from build123d import *

# Parameters (mm, degrees)
BOSS_EXTRUDE1_DEPTH       = 18
F_5_0MM_DOWEL_HOLE1_D     = 5
F_5_0MM_DOWEL_HOLE1_DEPTH = 3
F_5_0MM_DOWEL_HOLE1_TIP   = 1.502151548
FILLET1_R                 = 5
M3_CLEARANCE_HOLE1_D      = 3.6


with BuildPart() as part:
    # Sketch1 → Boss-Extrude1 (new body)
    with BuildSketch(Plane(origin=(0, 0, 0), x_dir=(0, 0, -1), z_dir=(1, 0, 0))):
        Polygon((0, 0), (28.1, 0), (28.1, 3), (3, 3), (3, 13), (0, 13), align=None)
    extrude(amount=BOSS_EXTRUDE1_DEPTH)

    # Ø5.0mm Dowel Hole1
    with Locations(Plane.XY):
        with Locations((9, 8)):
            Hole(F_5_0MM_DOWEL_HOLE1_D / 2, depth=F_5_0MM_DOWEL_HOLE1_DEPTH)
            with Locations((0, 0, -(F_5_0MM_DOWEL_HOLE1_DEPTH + F_5_0MM_DOWEL_HOLE1_TIP / 2))):  # 118° drill point
                Cone(0, F_5_0MM_DOWEL_HOLE1_D / 2, F_5_0MM_DOWEL_HOLE1_TIP, mode=Mode.SUBTRACT)

    # Fillet1
    fillet1_edges = [part.edges().sort_by_distance(p)[0] for p in [
        (18, 13, -1.5),
        (0, 13, -1.5),
    ]]
    fillet(fillet1_edges, radius=FILLET1_R)

    # M3 Clearance Hole1 (through all)
    with Locations(Plane(origin=(0, 3, 0), x_dir=(1, 0, 0), z_dir=(0, 1, 0))):
        with Locations((14, 24.6), (4, 24.6), (4, 14.6), (14, 14.6)):
            Hole(M3_CLEARANCE_HOLE1_D / 2)


solid = part.part
Work out the finished part from the listing and answer in its coordinate system (mm). A direction names the side the tool comes from. Coordinates: 2 decimals unless noted, no trailing zeros. Write each loop counter-clockwise with the first axis right and the second up, starting at its lowest first coordinate (ties: lowest second). Pieces come first, ordered by that corner, then holes. Notation, with made-up numbers: M 30.5,-29.5 L 86.5,-29.5 A14 cw 86.5,-8.5 Z; hole C 74,2 d4. An arc over 180 degrees is marked long. Use one line per item in the form item = value. Start each with the question number.
1. Each of these flat-tipped pins is pushed along its axis until it touches: P1, Ø5, axis at x = 7.5, y = 10.5, coming from the -Z side; P2, Ø2, axis at x = 13.5, z = -24.5, coming from the +Y side; P3, Ø6, axis at x = 14, z = -7.5, coming from the +Y side. Where does it stop, or does it pass through?
2. A tool of negligible diameter and unlimited length cuts with its end or side. For faces 1 (the face through (9, 3, -16)), 2 (the face through (18, 2, -11)), from which of +Z, -Z, +X, -X, +Y, -Y can it reach the whole face along a straight path? Write none if from no direction.
3. The mould has two halves that part along X. Classify faces 3 (the face through (3.169, 1.479, -23.003)), 4 (the face through (2, 12, -1)), 5 (the face through (9, 0, -14)): released by +X, released by -X, zero draft, split by the parting line, or undercut.
4. The part is cut by section C-C (x = 4). Give the vertices of the cut face in (y, z).
5. The part is cut by section D-D (y = 3.5). Give the vertices of the cut face in (x, z).
6. The part is cut by section B-B (x = 9). Give the vertices of the cut face in (y, z).
7. The part is cut by section A-A (z = -24.6). Give the vertices of the cut face in (x, y), plus the area to 3 significant figures.
8. Straight lines are drawn through the part: probe 1 along Z at (x, y) = (14, 0.65); probe 2 along X at (y, z) = (1.5, -24.6); probe 3 along Y at (x, z) = (13.25, -7). For each, find the intervals that lie inside material, in ascending order. Write a range as from..to.
Evaluation:
q1.P1 = -3
q1.P2 = through
q1.P3 = 3
q2.face_1 = -Z, +X, -X, +Y
q2.face_2 = +Z, -Z, +X, +Y, -Y
q3.face_3 = undercut
q3.face_4 = released by -X
q3.face_5 = zero draft
q4.outline = M 0,-28.1 L 3,-28.1 L 3,-26.4 L 0,-26.4 Z; M 0,-22.8 L 3,-22.8 L 3,-16.4 L 0,-16.4 Z; M 0,-12.8 L 3,-12.8 L 3,-3 L 12.9,-3 L 12.9,0 L 0,0 Z
q5.outline = M 0,-3 L 18,-3 L 18,0 L 0,0 Z
q6.outline = M 0,-28.1 L 3,-28.1 L 3,-3 L 5.5,-3 L 5.5,0 L 0,0 Z; M 10.5,-3 L 13,-3 L 13,0 L 10.5,0 Z
q7.outline = M 0,0 L 2.2,0 L 2.2,3 L 0,3 Z; M 5.8,0 L 12.2,0 L 12.2,3 L 5.8,3 Z; M 15.8,0 L 18,0 L 18,3 L 15.8,3 Z
q7.area = 32.4 mm^2
q8.probe_1 = -28.1..-26.4, -22.8..-16.4, -12.8..0
q8.probe_2 = 0..2.2, 5.8..12.2, 15.8..18
q8.probe_3 = 0..3
